Can you work these out from the drawing? Everything is in mm from the part's minimum corner. A direction names the side the tool comes from. Coordinates: 2 decimals unless noted, no trailing zeros. Loops run counter-clockwise (first coordinate to the right, second up) from the corner with the lowest first, then second, coordinate; pieces in that order, holes last. Notation, with made-up numbers: (58, -37.5) - (115, -37.5) arc R22 cw to (115, -21.5) - close; hole circle Ø9 at (-23, -30.5). An arc over 180 degrees is marked (long way). Put each result on its own line as item: value. Start each with the question number.
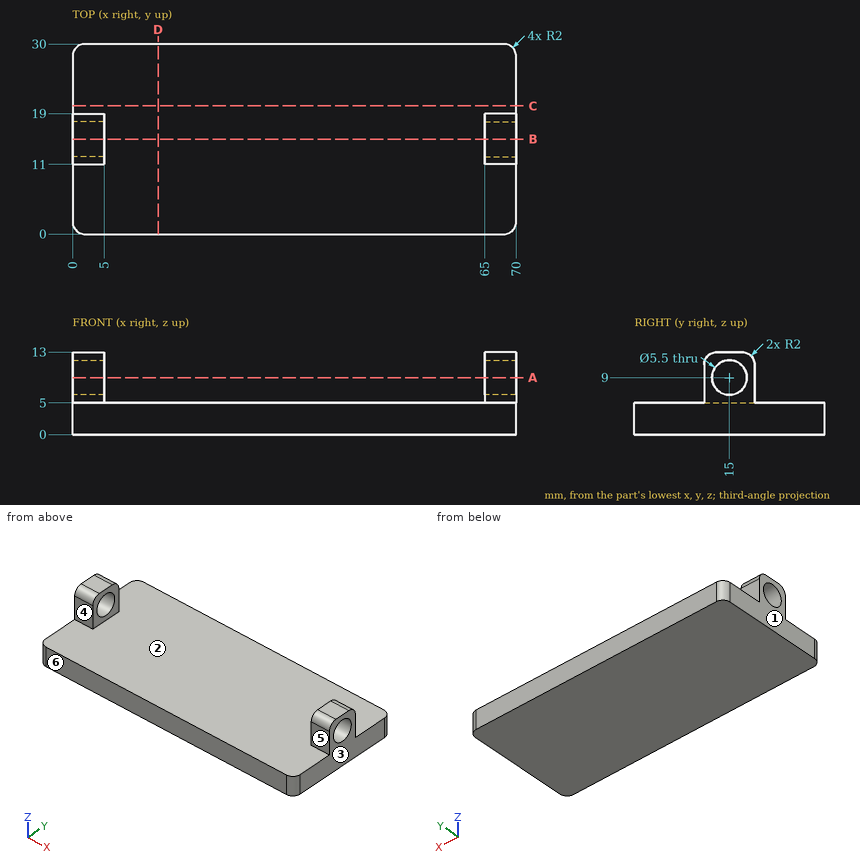
(1) I want a section at D-D on x = 13.5. List the corners of the cut face in (y, z) for me, and give its area (3 significant figures).
(2) I want a section at C-C on y = 20.25. List the corners of the cut face in (x, z) for me, and give its area (3 significant figures).
(3) I need wall thicknesses on L1, parallel to Y at x = 66.2, z = 9; L2, parallel to Z at x = 39.5, y = 19.25. Which ranges of each line are inside material? Lowest first, please. Write a range as [from, to].
(4) For pin 1 Ø5.5 at (x, z) = (2, 9) entering from -Y; pin 2 Ø2.5 at (x, z) = (68.5, 7) entering from +Y; pin 3 Ø15 at (x, y) = (20, 12) entering from +Z, each with a flat end and sliding along its axis, tell me the tip position at first contact or that it passes through.
(5) If we mould it in two halves opening along X, with no side actions, what happens to the marked faces 1, 2, 3 and 4? For each: pulls with the +X half, pulls with the -X half, needs draft (parallel to the pull), parting line crosses it, or undercut.
(6) I want a section at B-B on y = 15. List the corners of the cut face in (x, z) for me, and give its area (3 significant figures).
(7) Which directions (+Z, -Z, +X, -X, +Y, -Y) give clear straight access to the entire face, cutting with the end or side of a thin tool? Please do the marked faces 5 and 6.
(8) I want a section at A-A on z = 9. List the corners of the cut face in (x, y) for me, and give its area (3 significant figures).
Answer sheet:
1. outline: (0, 0) - (30, 0) - (30, 5) - (0, 5) - close
1. area: 150 mm^2
2. outline: (0, 0) - (70, 0) - (70, 5) - (0, 5) - close
2. area: 350 mm^2
3. L1: y = [11, 12.25], [17.75, 19]
3. L2: z = [0, 5]
4. pin 1: stops at y = 11
4. pin 2: stops at y = 19
4. pin 3: stops at z = 5
5. face 1: pulls with the -X half
5. face 2: undercut
5. face 3: pulls with the +X half
5. face 4: needs draft
6. outline: (0, 0) - (70, 0) - (70, 6.25) - (65, 6.25) - (65, 5) - (5, 5) - (5, 6.25) - (0, 6.25) - close; (0, 11.75) - (5, 11.75) - (5, 13) - (0, 13) - close; (65, 11.75) - (70, 11.75) - (70, 13) - (65, 13) - close
6. area: 375 mm^2
7. face 5: +Z, +X, -X, -Y
7. face 6: +Z, -Z, +X, -X, -Y
8. outline: (0, 11) - (5, 11) - (5, 12.25) - (0, 12.25) - close; (0, 17.75) - (5, 17.75) - (5, 19) - (0, 19) - close; (65, 11) - (70, 11) - (70, 12.25) - (65, 12.25) - close; (65, 17.75) - (70, 17.75) - (70, 19) - (65, 19) - close
8. area: 25.0 mm^2
